Could you check a few things on this drawing? It's one solid part, dimensions in mm from its lowest x, y, z. Give positions to 0.01 mm unless a question says otherwise; leave off trailing zeros. Order: outer loops, then holes, each group sorted by start corner. A loop starts at its lowest first (then second) coordinate and runs counter-clockwise, first axis right, second up. Notation, with made-up numbers: (47.25, -20) - (73.25, -20) arc R23 cw to (73.25, 1) - close; hole circle Ø9 at (-23.5, -31.75). An arc over 180 degrees is marked (long way). Return JSON: item names as keys, results as strings.
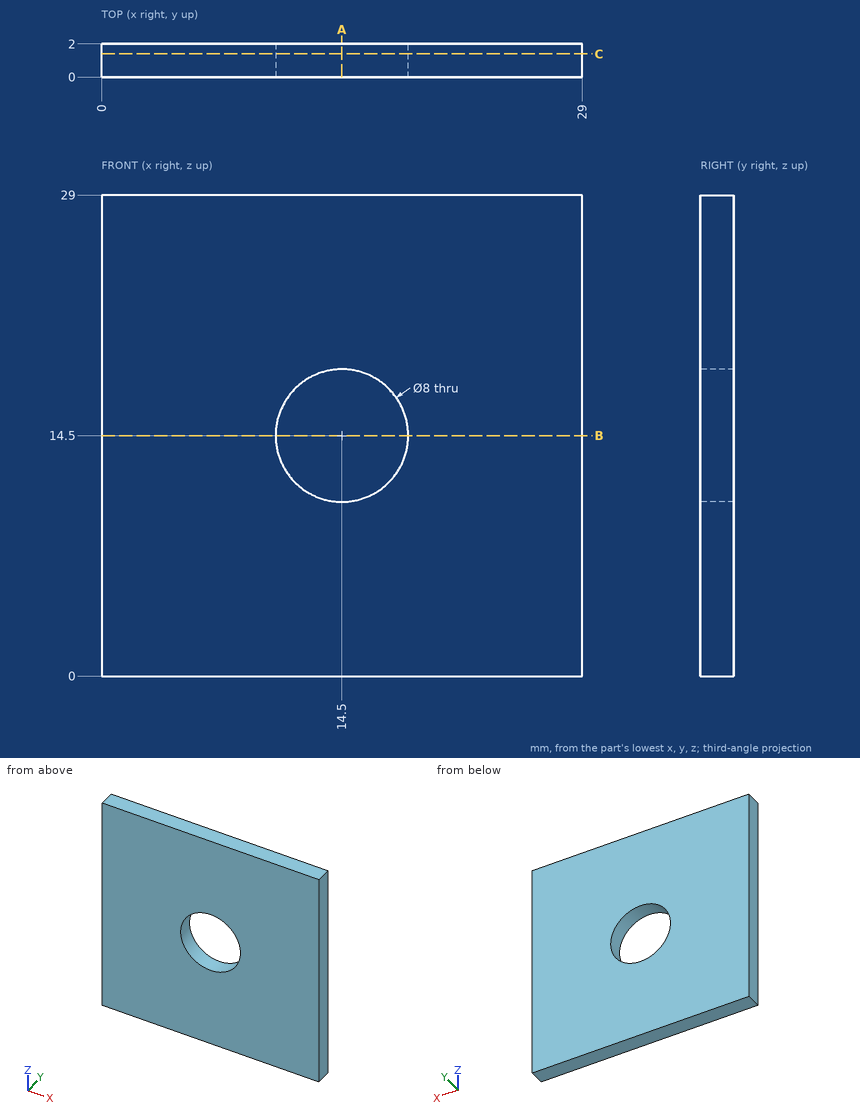
1. Suppose I cut it at A-A (x = 14.5). List the corners of the cut face in (y, z) for me.
Checks:
{"outline": "(0, 0) - (2, 0) - (2, 10.5) - (0, 10.5) - close; (0, 18.5) - (2, 18.5) - (2, 29) - (0, 29) - close"}
2. Suppose I cut it at C-C (y = 1.4). List the corners of the cut face in (x, z) for me, plus the area to 3 significant figures.
Checks:
{"outline": "(0, 0) - (29, 0) - (29, 29) - (0, 29) - close; hole circle Ø8 at (14.5, 14.5)", "area": "791 mm^2"}
3. If I drill on L1, parallel to Z at x = 14.5, y = 1.1; L2, parallel to X at y = 0.6, z = 15; L3, parallel to Z at x = 15.75, y = 0.3, over which ranges is the centre line in solid material (lowest first)? Write a range as [from, to].
Checks:
{"L1": "[0, 10.5], [18.5, 29]", "L2": "[0, 10.53], [18.47, 29]", "L3": "[0, 10.7], [18.3, 29]"}
4. Suppose I cut it at B-B (z = 14.5). List the corners of the cut face in (x, y) for me.
Checks:
{"outline": "(0, 0) - (10.5, 0) - (10.5, 2) - (0, 2) - close; (18.5, 0) - (29, 0) - (29, 2) - (18.5, 2) - close"}
